For this review, take the finished solid that the model builds, in its own axes (mm). A direction names the side the tool comes from. Coordinates: 2 decimals unless noted, no trailing zeros. Write each loop counter-clockwise with the first axis right and the second up, starting at its lowest first coordinate (ties: lowest second). Pieces come first, ordered by that corner, then holes.
1) We need section C-C on y = 3.85. Write out the cut boundary in (x, z), then the cut area to 3 significant figures.
2) For faces 4 (the face through (22, 2, 56.1)), 5 (the face through (1.348, 2, 54)), 6 (the face through (20, 2, 21)), list the 3-axis set-ups (+Z, -Z, +X, -X, +Y, -Y) from which the entire face can be reached by the end or side of a thin tool; tool diameter is ignored.
3) Mouldability with a two-part tool opening along X and no side actions: class faces 1 (the face through (10, 2, 0)), 2 (the face through (-1, 2, 56.205)), 3 (the face through (-4.25, 2, 23)) as pulls with the +X half, pulls with the -X half, needs draft (parallel to the pull), parting line crosses it, or undercut.
4) To check wall thickness, follow line 1 along X through (y, z) = (1.95, -4); line 2 along X through (y, z) = (3.85, 18.5); line 3 along Z through (x, y) = (4.75, 1.05). State the ranges of each line that lie inside material, in increasing order.
5) We need section D-D on z = -4. Write out the cut boundary in (x, y).
6) We need section A-A on x = 8.5. Write out the cut boundary in (y, z), then the cut area to 3 significant figures.
7) We need section B-B on z = 38.5. Write out the cut boundary in (x, y).
8) Insertion check: P1, Ø2.5, axis at x = 5, z = -4, coming from the -Y side; P2, Ø1.5, axis at x = 14, y = 2.5, coming from the +Z side; P3, Ø2.5, axis at x = 23, y = 3, coming from the +Z side. Each pin has a flat end and moves straight along its axis. Give the tip position at first contact, or say it passes through.
from build123d import *

# Parameters (mm, degrees)
SKETCH1_R           = 2.25
SKETCH1_W           = 20
SKETCH1_H           = 40.6
BOSS_EXTRUDE1_DEPTH = 5


with BuildPart() as part:
    # Sketch1 → Boss-Extrude1 (new body)
    with BuildSketch(Plane(origin=(0, 0, 0), x_dir=(1, 0, 0), z_dir=(0, 1, 0))):
        Polygon((-4.25, -48), (-4.25, 7.4), (-4.25, 9.9), (24.25, 9.9), (24.25, 7.4), (24.25, -48), (24.25, -56.1), (18.848117926, -56.1), (18.848117926, -51.1), (1.348117926, -51.1), (1.348117926, -56.204802146), (-4.25, -56.204802146), align=None)
        with Locations(Location((5, 4, 0), (0, 0, 270))):
            Circle(SKETCH1_R, mode=Mode.SUBTRACT)
        with Locations(Location((15, 4, 0), (0, 0, 90))):
            Circle(SKETCH1_R, mode=Mode.SUBTRACT)
        with Locations(Location((5, -44.6, 0), (0, 0, 90))):
            Circle(SKETCH1_R, mode=Mode.SUBTRACT)
        with Locations(Location((15, -44.6, 0), (0, 0, 270))):
            Circle(SKETCH1_R, mode=Mode.SUBTRACT)
        with Locations((10, -20.3)):
            Rectangle(SKETCH1_W, SKETCH1_H, mode=Mode.SUBTRACT)
    extrude(amount=BOSS_EXTRUDE1_DEPTH)


solid = part.part
Result:
1. outline: (-4.25, -9.9) - (24.25, -9.9) - (24.25, 56.1) - (18.85, 56.1) - (18.85, 51.1) - (1.35, 51.1) - (1.35, 56.2) - (-4.25, 56.2) - close; hole (0, 0) - (20, 0) - (20, 40.6) - (0, 40.6) - close; hole circle Ø4.5 at (5, -4); hole circle Ø4.5 at (5, 44.6); hole circle Ø4.5 at (15, -4); hole circle Ø4.5 at (15, 44.6)
1. area: 918 mm2
2. face 4: +Z, +X, +Y, -Y
2. face 5: +Z, +Y, -Y
2. face 6: +Y, -Y
3. face 1: undercut
3. face 2: needs draft
3. face 3: pulls with the -X half
4. line 1: x = -4.25 to 2.75, 7.25 to 12.75, 17.25 to 24.25
4. line 2: x = -4.25 to 0, 20 to 24.25
4. line 3: z = -9.9 to -6.24, -1.76 to 0, 40.6 to 42.36, 46.84 to 51.1
5. outline: (-4.25, 0) - (2.75, 0) - (2.75, 5) - (-4.25, 5) - close; (7.25, 0) - (12.75, 0) - (12.75, 5) - (7.25, 5) - close; (17.25, 0) - (24.25, 0) - (24.25, 5) - (17.25, 5) - close
6. outline: (0, -9.9) - (5, -9.9) - (5, 0) - (0, 0) - close; (0, 40.6) - (5, 40.6) - (5, 51.1) - (0, 51.1) - close
6. area: 102 mm2
7. outline: (-4.25, 0) - (0, 0) - (0, 5) - (-4.25, 5) - close; (20, 0) - (24.25, 0) - (24.25, 5) - (20, 5) - close
8. P1: passes through
8. P2: stops at z = 51.1
8. P3: stops at z = 56.1
